Part print with two shaded views. Sizes in mm from the minimum x, y, z corner. Coordinates: 2 decimals unless noted, no trailing zeros. Order: outer loops, then holes, each group sorted by start corner. A loop starts at its lowest first (then second) coordinate and runs counter-clockwise, first axis right, second up. Notation, with made-up numbers: (57, 65) - (70, 65) arc R16 cw to (70, 96) - close; hole circle Ø3 at (35.25, 34.5). An arc over 180 degrees is marked (long way). Write each question's results on one line, items separated by ' | '. Start each with the question number.
Q1. Band-saw the part on C-C, the plane x = 36. Write the cut outline in (y, z) (1 decimal), then the cut area to 3 significant figures.
Q2. Pull direction X, two halves, no side cores. Call the marked faces 1, 2 and 3: released by +X, released by -X, zero draft, split by the parting line, or undercut.
Q3. Band-saw the part on B-B, the plane x = 91.44. Write the cut outline in (y, z).
Q4. Pin check, flat tips, straight feed: P1, Ø3, axis at y = 71.5, z = 153, coming from the +X side; P2, Ø1, axis at x = 87, y = 40, coming from the +Z side. Stop position of each tip, or through.
Q5. Band-saw the part on D-D, the plane y = 92. Write the cut outline in (x, z), then the cut area to 3 significant figures.
Q6. Wall check: probe 1 along Z at (x, y) = (145.5, 73.5); probe 2 along X at (y, z) = (78.5, 126) (1 decimal); probe 3 along Y at (x, z) = (99.5, 61) (1 decimal). Give the ranges that are in metal, low to high.
Q7. Band-saw the part on A-A, the plane x = 62. Count the separate pieces of the cut face and the enclosed holes in it, then the cut area to 3 significant figures.
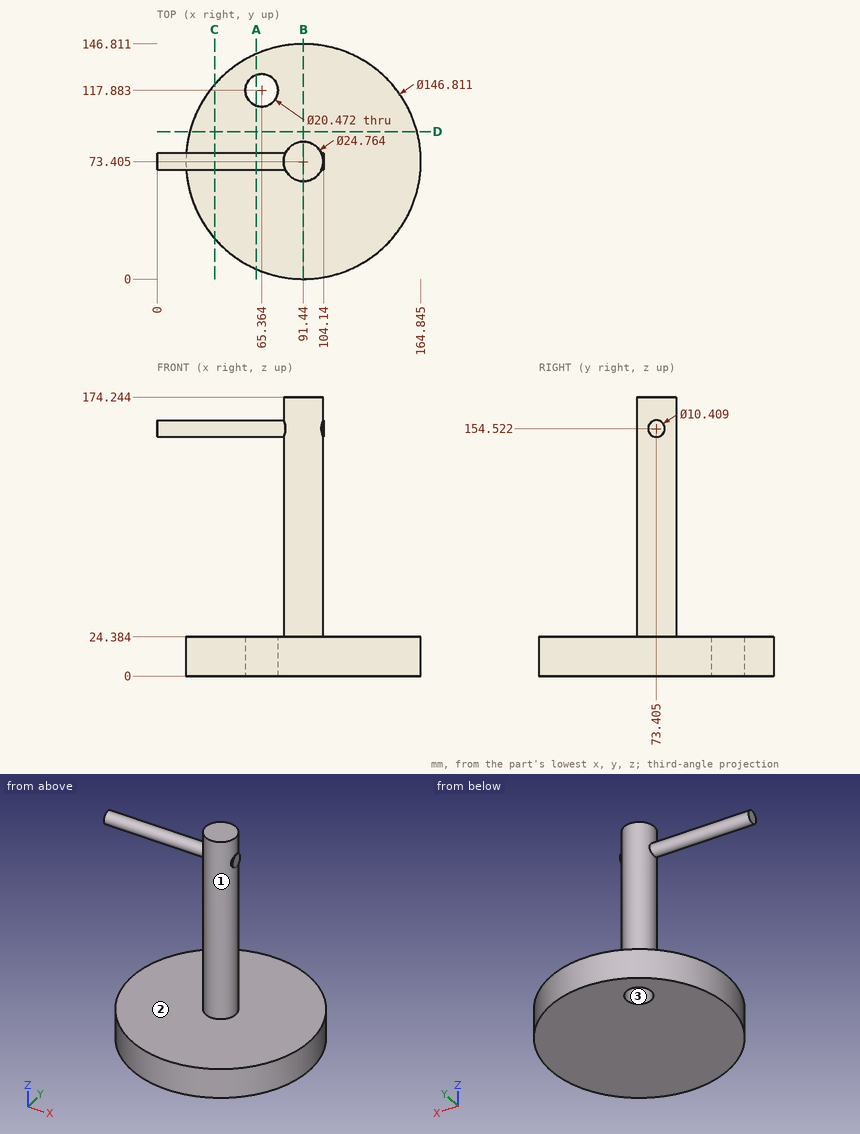
Results below:
1) outline: (25.3, 0) - (121.5, 0) - (121.5, 24.4) - (25.3, 24.4) - close; circle Ø10.4 at (73.4, 154.5) | area: 2,430 mm²
2) face 1: split by the parting line | face 2: zero draft | face 3: undercut
3) outline: (0, 0) - (146.81, 0) - (146.81, 24.38) - (85.79, 24.38) - (85.79, 174.24) - (61.02, 174.24) - (61.02, 24.38) - (0, 24.38) - close
4) P1: stops at x = 104.14 | P2: stops at z = 24.38
5) outline: (20.43, 0) - (162.45, 0) - (162.45, 24.38) - (20.43, 24.38) - close | area: 3,460 mm²
6) probe 1: z = 0 to 24.38 | probe 2: x = 80.2 to 102.7 | probe 3: y = 64 to 82.8
7) separate pieces: 3 | enclosed holes: 0 | area: 2,890 mm²
